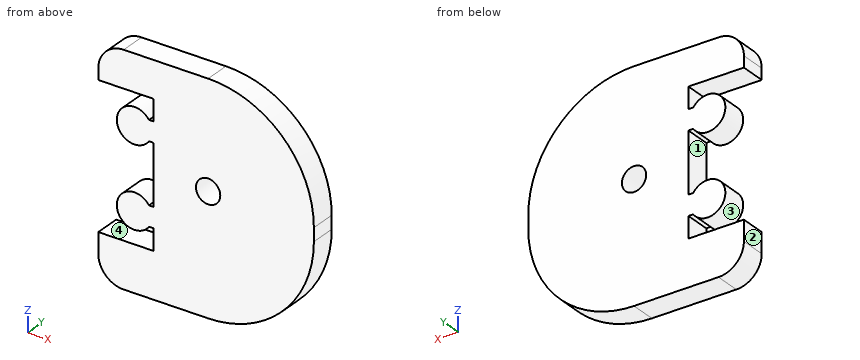
from build123d import *

# Parameters (mm, degrees)
SKETCH1_W           = 50.8
SKETCH1_H           = 21.59
BOSS_EXTRUDE1_DEPTH = 3.175
FILLET1_R           = 10.16
SKETCH3_R           = 1.16713
CUT_EXTRUDE1_DEPTH  = 28.780796425
FILLET3_R           = 10.16
SCALE1_SCALE_X      = 1.3
SCALE1_SCALE_Y      = 1
SCALE1_SCALE_Z      = 1.3
SKETCH4_W           = 39.116
SKETCH4_H           = 28.067
CUT_EXTRUDE2_DEPTH  = 37.032702199
CUT_EXTRUDE3_DEPTH  = 37.032702199
FILLET5_R           = 3.175


with BuildPart() as part:
    # Sketch1 → Boss-Extrude1 (new body)
    with BuildSketch(Plane(origin=(0, 0, 0), x_dir=(1, 0, 0), z_dir=(0, 1, 0))):
        Rectangle(SKETCH1_W, SKETCH1_H)
    extrude(amount=BOSS_EXTRUDE1_DEPTH)

    # Fillet1
    fillet1_edges = [part.edges().sort_by_distance(p)[0] for p in [
        (25.4, 1.5875, 10.795),
        (-25.4, 1.5875, 10.795),
    ]]
    fillet(fillet1_edges, radius=FILLET1_R)

    # Sketch3 → Cut-Extrude1 (cut, through all)
    with BuildSketch(Plane(origin=(0, 3.175, 0), x_dir=(1, 0, 0), z_dir=(0, 1, 0))):
        with Locations(Location((15.24, -0.635, 0), (0, 0, 270))):
            Circle(SKETCH3_R)
        with Locations(Location((-3.81, -0.635, 0), (0, 0, 270))):
            Circle(SKETCH3_R)
    extrude(amount=-CUT_EXTRUDE1_DEPTH, mode=Mode.SUBTRACT)

    # Fillet3
    fillet3_edges = [part.edges().sort_by_distance(p)[0] for p in [
        (-25.4, 1.5875, -10.795),
        (25.4, 1.5875, -10.795),
    ]]
    fillet(fillet3_edges, radius=FILLET3_R)


with BuildPart() as part_1:
    # Scale1: scaled about (-0.04893356, 1.5875, -0.005437062)
    add(part.part.scale((SCALE1_SCALE_X, SCALE1_SCALE_Y, SCALE1_SCALE_Z), about=(-0.04893356, 1.5875, -0.005437062)))

    # Sketch4 → Cut-Extrude2 (cut, through all)
    with BuildSketch(Plane(origin=(0, 3.175, 0), x_dir=(1, 0, 0), z_dir=(0, 1, 0))):
        with Locations((-13.447319932, -0.001631119)):
            Rectangle(SKETCH4_W, SKETCH4_H)
    extrude(amount=-CUT_EXTRUDE2_DEPTH, mode=Mode.SUBTRACT)

    # Sketch5 → Cut-Extrude3 (cut, through all)
    with BuildSketch(Plane(origin=(0, 3.175, 0), x_dir=(1, 0, 0), z_dir=(0, 1, 0))):
        with BuildLine():
            Line((13.035792068, -6.830615627), (13.035792068, -9.480615627))
            Line((13.035792068, -9.480615627), (6.110680068, -9.480615627))
            Line((6.110680068, -9.480615627), (6.110680068, 8.319384373))
            Line((6.110680068, 8.319384373), (13.035792068, 8.319384373))
            Line((13.035792068, 8.319384373), (13.035792068, 5.669384373))
            Line((13.035792068, 5.669384373), (12.435792068, 5.669384373))
            ThreePointArc((12.435792068, 5.669384373), (8.425405369, 4.419384373), (12.435792068, 3.169384373))
            Line((12.435792068, 3.169384373), (13.035792068, 3.169384373))
            Line((13.035792068, 3.169384373), (13.035792068, -4.330615627))
            Line((13.035792068, -4.330615627), (12.435792068, -4.330615627))
            ThreePointArc((12.435792068, -4.330615627), (8.425405369, -5.580615627), (12.435792068, -6.830615627))
            Line((12.435792068, -6.830615627), (13.035792068, -6.830615627))
        make_face()
    extrude(amount=-CUT_EXTRUDE3_DEPTH, mode=Mode.SUBTRACT)

    # Fillet5
    fillet5_edges = [part_1.edges().sort_by_distance(p)[0] for p in [
        (6.110680068, 1.5875, -14.031868881),
        (6.110680068, 1.5875, 14.035131119),
    ]]
    fillet(fillet5_edges, radius=FILLET5_R)


solid = part_1.part
For this review, take the finished solid that the model builds, in its own axes (mm). Face numbers are marked on the shaded views. A direction names the side the tool comes from. Give positions to 0.01 mm unless a question says otherwise; leave off trailing zeros. Answer as a JSON object with one key per item and string values. Group by question number.
Q1. Tool access review of the marked faces 3 and 4: name each direction out of +Z, -Z, +X, -X, +Y, -Y from which nothing blocks a thin tool from reaching the whole face with its end or side.
Q2. Add section A-A on x = 11.75. Give the number of separate pieces and of enclosed holes in the cut face, and give its area (3 significant figures).
Q3. Insertion check: P1, Ø1.5, axis at x = 30, y = 2, coming from the +Z side; P2, Ø1.6, axis at y = 1.5, z = 1.5, coming from the -X side; P3, Ø1, axis at y = 2, z = -3.5, coming from the +X side. Each pin has a flat end and moves straight along its axis. Give the tip position at first contact, or say it passes through.
Q4. For probe 1 along Z at (x, y) = (10.5, 0.45); probe 2 along Z at (x, y) = (11.5, 2.45); probe 3 along X at (y, z) = (1.3, 0.75), list the stretches that pass through material, from the lowest coordinate up. Write a range as [from, to].
Q5. Mouldability with a two-part tool opening along Z and no side actions: class the marked faces 1 and 2 as +Z half, -Z half, draft (parallel to the pull), parting line (faces both ways), or undercut.
Checked values:
{
 "1": {"face 3": "+Y, -Y", "face 4": "-X, +Y, -Y"},
 "2": {"separate pieces": "4", "enclosed holes": "0", "area": "56.6 mm²"},
 "3": {"P1": "z = 10.08", "P2": "x = 13.04", "P3": "x = 32.85"},
 "4": {"probe 1": "[-14.03, -8.32], [-6.62, -2.22], [3.38, 7.78], [9.48, 14.04]", "probe 2": "[-14.03, -8.32], [-6.44, -2.4], [3.56, 7.6], [9.48, 14.04]", "probe 3": "[13.04, 18.31], [21.34, 33.03]"},
 "5": {"face 1": "undercut", "face 2": "draft"}
}
